```python
from build123d import *

# Parameters (mm, degrees)
F0_W        = 90
F0_H        = 38
F1_DEPTH    = 2.5
F3_D        = 3.4
F2_W        = 35.7
F2_H        = 38
F4_DEPTH    = 3
F6_W        = 23.7
F6_H        = 26
F5_W        = 23.7
F5_H        = 26
F7_DEPTH    = 10
F10_D       = 2.9
F10_ON_F9_D = 2.9
F11_R       = 3


with BuildPart() as f1:
    # F0 (on Top) → F1 (new body)
    with BuildSketch(Plane.XY):
        Rectangle(F0_W, F0_H)
    extrude(amount=F1_DEPTH)

    # F3 (through all)
    with Locations(Plane.XY.offset(2.5)):
        with Locations((6.625, -14.7051038221), (-6.625, -14.7051038221)):
            Hole(F3_D / 2)

    # F2 (on face) → F4 (join)
    with BuildSketch(Plane.XY.offset(2.5)):
        with Locations((-27.15, 0)):
            Rectangle(F2_W, F2_H)
        with Locations((27.15, 0)):
            Rectangle(F2_W, F2_H)
    extrude(amount=F4_DEPTH)

    # F6 (on face) + F5 (on face) → F7 (cut)
    with BuildSketch(Plane.XY.offset(5.5)):
        with Locations((-27.15, 0)):
            Rectangle(F6_W, F6_H)
    with BuildSketch(Plane.XY.offset(5.5)):
        with Locations((27.15, 0)):
            Rectangle(F5_W, F5_H)
    extrude(amount=-F7_DEPTH, mode=Mode.SUBTRACT)

    # F10 (through all)
    with Locations(Plane.XY.offset(5.5)):
        with Locations((-41.2, 15.2), (-41.2, -15.3), (-13.1, 15.2), (-13.1, -15.3)):
            Hole(F10_D / 2)

    # F10 on F9 (through all)
    with Locations(Plane.XY.offset(5.5)):
        with Locations((13.1, 15.2), (41.2, 15.2), (13.1, -15.3), (41.2, -15.3)):
            Hole(F10_ON_F9_D / 2)

    # F11
    f11_edges = [f1.edges().sort_by_distance(p)[0] for p in [
        (-45, 19, 2.75),
        (9.3, 19, 4),
        (45, 19, 2.75),
        (39, -13, 2.75),
        (-15.3, -13, 2.75),
        (-45, -19, 2.75),
        (-9.3, -19, 4),
        (-39, 13, 2.75),
        (-9.3, 19, 4),
        (15.3, 13, 2.75),
        (45, -19, 2.75),
        (15.3, -13, 2.75),
        (-39, -13, 2.75),
        (-15.3, 13, 2.75),
        (39, 13, 2.75),
        (9.3, -19, 4),
    ]]
    fillet(f11_edges, radius=F11_R)


solid = f1.part
```
For this review, take the finished solid that the model builds, in its own axes (mm). A direction names the side the tool comes from. Give positions to 0.01 mm unless a question says otherwise; leave off trailing zeros. Order: outer loops, then holes, each group sorted by start corner. A loop starts at its lowest first (then second) coordinate and runs counter-clockwise, first axis right, second up.
1) Take a section at A-A (x = 31). Give the boundary of the cut face in (y, z), then the cut area to 3 significant figures.
2) Take a section at D-D (y = 15.2). Give the boundary of the cut face in (x, z), then the cut area to 3 significant figures.
3) Wall thickness on line 1 (Y direction, x = 13.1, z = 1.3); line 2 (X direction, y = 8, z = 3.5); line 3 (X direction, y = -4, z = 0.3): over which ranges is each line inside the solid? List them lowest first.
4) Take a section at C-C (x = 13.1). Give the boundary of the cut face in (y, z), then the cut area to 3 significant figures.
5) For faces 5 (the face through (-38.1, -12.14, 2.71)), 6 (the face through (-10.2, -18.14, 4.02)), 7 (the face through (-9.3, 0, 4)), 8 (the face through (10.2, 18.14, 4.02)), list the 3-axis set-ups (+Z, -Z, +X, -X, +Y, -Y) from which the entire face can be reached by the end or side of a thin tool; tool diameter is ignored.
6) The part is to be moulded in two halves that separate along Y. For faces 1 (the face through (10.2, -18.14, 4.02)), 2 (the face through (-16.16, 12.1, 2.71)), 3 (the face through (-10.2, 18.14, 4.02)), 4 (the face through (0, 0, 2.5)), say which applies: released by +Y, released by -Y, zero draft, split by the parting line, or undercut.
7) Take a section at B-B (y = -3). Give the boundary of the cut face in (x, z), then the cut area to 4 significant figures.
Derived:
1. outline: (-19, 0) - (-13, 0) - (-13, 5.5) - (-19, 5.5) - close; (13, 0) - (19, 0) - (19, 5.5) - (13, 5.5) - close
1. area: 66.0 mm2
2. outline: (-45, 0) - (-42.65, 0) - (-42.65, 5.5) - (-45, 5.5) - close; (-39.75, 0) - (-14.55, 0) - (-14.55, 5.5) - (-39.75, 5.5) - close; (-11.65, 0) - (11.65, 0) - (11.65, 5.5) - (9.3, 5.5) - (9.3, 2.5) - (-9.3, 2.5) - (-9.3, 5.5) - (-11.65, 5.5) - close; (14.55, 0) - (39.75, 0) - (39.75, 5.5) - (14.55, 5.5) - close; (42.65, 0) - (45, 0) - (45, 5.5) - (42.65, 5.5) - close
2. area: 375 mm2
3. line 1: y = -19 to -16.75, -13.85 to 13.75, 16.65 to 19
3. line 2: x = -45 to -39, -15.3 to -9.3, 9.3 to 15.3, 39 to 45
3. line 3: x = -45 to -39, -15.3 to 15.3, 39 to 45
4. outline: (-19, 0) - (-16.75, 0) - (-16.75, 5.5) - (-19, 5.5) - close; (-13.85, 0) - (13.75, 0) - (13.75, 5.5) - (-13.85, 5.5) - close; (16.65, 0) - (19, 0) - (19, 5.5) - (16.65, 5.5) - close
4. area: 177 mm2
5. face 5: +Z, -Z
5. face 6: +Z, -Y
5. face 7: +Z, +Y, -Y
5. face 8: +Z, +Y
6. face 1: released by -Y
6. face 2: undercut
6. face 3: released by +Y
6. face 4: zero draft
7. outline: (-45, 0) - (-39, 0) - (-39, 5.5) - (-45, 5.5) - close; (-15.3, 0) - (15.3, 0) - (15.3, 5.5) - (9.3, 5.5) - (9.3, 2.5) - (-9.3, 2.5) - (-9.3, 5.5) - (-15.3, 5.5) - close; (39, 0) - (45, 0) - (45, 5.5) - (39, 5.5) - close
7. area: 178.5 mm2
